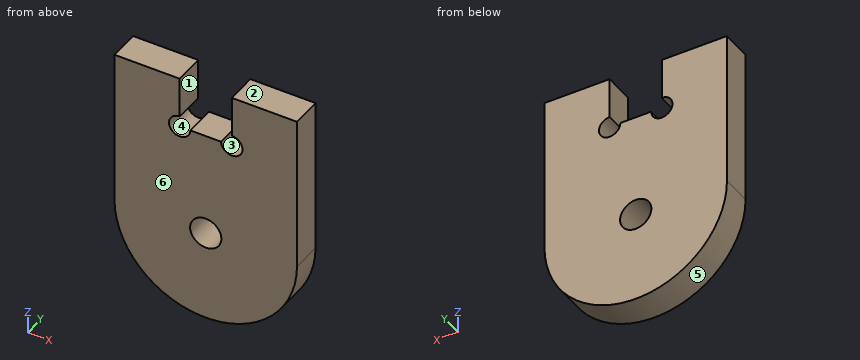
```python
from build123d import *

# Parameters (mm, degrees)
SKETCH1_R           = 3
BOSS_EXTRUDE1_DEPTH = 5.9
CUT_EXTRUDE1_REACH  = 7.9
SKETCH2_W           = 10
SKETCH2_H           = 11.8
SKETCH3_W           = 12.5
SKETCH3_H           = 5.9
BOSS_EXTRUDE2_DEPTH = 5
CUT_EXTRUDE2_REACH  = 7.9
SKETCH4_R           = 2.05


with BuildPart() as part:
    # Sketch1 → Boss-Extrude1 (new body)
    with BuildSketch(Plane(origin=(0, 0, 0), x_dir=(1, 0, 0), z_dir=(0, 1, 0))):
        with BuildLine():
            ThreePointArc((17.5, 12.5), (0, 30), (-17.5, 12.5))
            Line((-17.5, 12.5), (-17.5, -12.5))
            Line((-17.5, -12.5), (17.5, -12.5))
            Line((17.5, -12.5), (17.5, 12.5))
        make_face()
        with Locations((0, 12.5)):
            Circle(SKETCH1_R, mode=Mode.SUBTRACT)
    extrude(amount=BOSS_EXTRUDE1_DEPTH)

    # Sketch2 → Cut-Extrude1 (cut, up to next)
    with BuildSketch(Plane(origin=(0, 5.9, 0), x_dir=(1, 0, 0), z_dir=(0, 1, 0)), mode=Mode.PRIVATE) as cut_extrude1_sk1:
        with Locations((0, -13.5)):
            Rectangle(SKETCH2_W, SKETCH2_H)
    cut_extrude1_tool1 = extrude(cut_extrude1_sk1.sketch, amount=-CUT_EXTRUDE1_REACH, mode=Mode.PRIVATE) & part.part
    add(cut_extrude1_tool1.solids().sort_by_distance((0, 5.9, 13.5))[0], mode=Mode.SUBTRACT)

    # Sketch3 → Boss-Extrude2 (add)
    with BuildSketch(Plane.XY.offset(12.5)):
        with Locations((-11.25, 2.95)):
            Rectangle(SKETCH3_W, SKETCH3_H)
        with Locations((11.25, 2.95)):
            Rectangle(SKETCH3_W, SKETCH3_H)
    extrude(amount=BOSS_EXTRUDE2_DEPTH)

    # Sketch4 → Cut-Extrude2 (cut, up to next)
    with BuildSketch(Plane(origin=(0, 5.9, 0), x_dir=(1, 0, 0), z_dir=(0, 1, 0)), mode=Mode.PRIVATE) as cut_extrude2_sk1:
        with Locations((-5, -7.6)):
            Circle(SKETCH4_R)
    cut_extrude2_tool1 = extrude(cut_extrude2_sk1.sketch, amount=-CUT_EXTRUDE2_REACH, mode=Mode.PRIVATE) & part.part
    add(cut_extrude2_tool1.solids().sort_by_distance((-5, 5.9, 7.6))[0], mode=Mode.SUBTRACT)
    # Sketch4 → Cut-Extrude2 (cut, up to next)
    with BuildSketch(Plane(origin=(0, 5.9, 0), x_dir=(1, 0, 0), z_dir=(0, 1, 0)), mode=Mode.PRIVATE) as cut_extrude2_sk2:
        with Locations((5, -7.6)):
            Circle(SKETCH4_R)
    cut_extrude2_tool2 = extrude(cut_extrude2_sk2.sketch, amount=-CUT_EXTRUDE2_REACH, mode=Mode.PRIVATE) & part.part
    add(cut_extrude2_tool2.solids().sort_by_distance((5, 5.9, 7.6))[0], mode=Mode.SUBTRACT)


solid = part.part
```
Here's how the part is built. I have some questions about the finished solid (model axes, mm). Face numbers are marked on the shaded views. A direction names the side the tool comes from. Coordinates: 2 decimals unless noted, no trailing zeros. Order: outer loops, then holes, each group sorted by start corner. A loop starts at its lowest first (then second) coordinate and runs counter-clockwise, first axis right, second up.
1) Imagine slicing it at A-A on x = 0. List the corners of the cut face in (y, z) for me.
2) Imagine slicing it at B-B on y = 0.8. List the corners of the cut face in (x, z) for me, and give its area (3 significant figures).
3) Which directions (+Z, -Z, +X, -X, +Y, -Y) give clear straight access to the entire face, cutting with the end or side of a thin tool? Please do the marked faces 1 and 2.
4) Imagine slicing it at C-C on z = 7. List the corners of the cut face in (x, y) for me, and give its area (3 significant figures).
5) Imagine slicing it at D-D on z = -16.5. List the corners of the cut face in (x, y) for me, and give its area (3 significant figures).
6) I need wall thicknesses on line 1 (X direction, y = 0.85, z = -12.5); line 2 (X direction, y = 4, z = 12.5); line 3 (X direction, y = 4.65, z = 7). Which ranges of each line are inside material? Lowest first, please.
7) We'd pull the mould along Z, two halves only. Please class the marked faces 3, 4, 5 and 6: +Z half, -Z half, draft (parallel to the pull), parting line (faces both ways), or undercut.
8) Will these pins go through, and if not, where does the flat tip stop? pin 1 (3.5 mm diameter, centred on x = 5, z = 7.6, fed in from +Y); pin 2 (1.8 mm diameter, centred on x = -1, y = 2.5, fed in from +Z); pin 3 (1.5 mm diameter, centred on x = -10.5, y = 1.5, fed in from -Z); pin 4 (1 mm diameter, centred on x = 5.5, y = 1, fed in from -Z).
Response values:
1. outline: (0, -30) - (5.9, -30) - (5.9, -15.5) - (0, -15.5) - close; (0, -9.5) - (5.9, -9.5) - (5.9, 7.6) - (0, 7.6) - close
2. outline: (-17.5, -12.5) arc R17.5 ccw to (17.5, -12.5) - (17.5, 17.5) - (5, 17.5) - (5, 9.65) arc R2.05 cw (long way) to (2.95, 7.6) - (-2.95, 7.6) arc R2.05 cw (long way) to (-5, 9.65) - (-5, 17.5) - (-17.5, 17.5) - close; hole circle Ø6 at (0, -12.5)
2. area: 1,380 mm2
3. face 1: +Z, +Y, -Y
3. face 2: +Z, +X, -X, +Y, -Y
4. outline: (-17.5, 0) - (-6.96, 0) - (-6.96, 5.9) - (-17.5, 5.9) - close; (-3.04, 0) - (3.04, 0) - (3.04, 5.9) - (-3.04, 5.9) - close; (6.96, 0) - (17.5, 0) - (17.5, 5.9) - (6.96, 5.9) - close
4. area: 160 mm2
5. outline: (-17.04, 0) - (17.04, 0) - (17.04, 5.9) - (-17.04, 5.9) - close
5. area: 201 mm2
6. line 1: x = -17.5 to -3, 3 to 17.5
6. line 2: x = -17.5 to -5, 5 to 17.5
6. line 3: x = -17.5 to -6.96, -3.04 to 3.04, 6.96 to 17.5
7. face 3: undercut
7. face 4: undercut
7. face 5: -Z half
7. face 6: draft
8. pin 1: passes through
8. pin 2: stops at z = 7.6
8. pin 3: stops at z = -27.03
8. pin 4: stops at z = -29.27
